The drawing under review shows one solid part. Ordinate dimensions are in mm from its lowest x, y, z. Coordinates: 2 decimals unless noted, no trailing zeros. Write each loop counter-clockwise with the first axis right and the second up, starting at its lowest first coordinate (ties: lowest second). Pieces come first, ordered by that corner, then holes.
Q1. Add section B-B, the plane y = 81.5. Give the boundary of the cut face in (x, z), plus the area to 3 significant figures.
Q2. Add section A-A, the plane x = 61.5. Give the boundary of the cut face in (y, z).
Q3. The part is to be moulded in two halves that separate along Y. For the marked faces 1, 2 and 3, say which applies: +Y half, -Y half, draft (parallel to the pull), parting line (faces both ways), or undercut.
Q4. Add section C-C, the plane x = 92. Give the boundary of the cut face in (y, z) (1 decimal).
Q5. To check wall thickness, follow probe 1 along Y at (x, z) = (61.5, 7.55); probe 2 along X at (y, z) = (52.5, 1) (1 decimal); probe 3 along X at (y, z) = (23, 5.5) (1 decimal). State the ranges of each line that lie inside material, in increasing order.
Q6. Clearance check with flat-ended pins moving along their axes: pin 1 Ø2.5 at (x, y) = (61.5, 6) entering from +Z; pin 2 Ø4.5 at (y, z) = (62, 2.5) entering from -X; pin 3 Ø1 at (y, z) = (86, 1) entering from +X; pin 4 Ø5 at (y, z) = (94.5, 3) entering from +X (1 decimal). State where each tip first meets the part, or that it passes through.
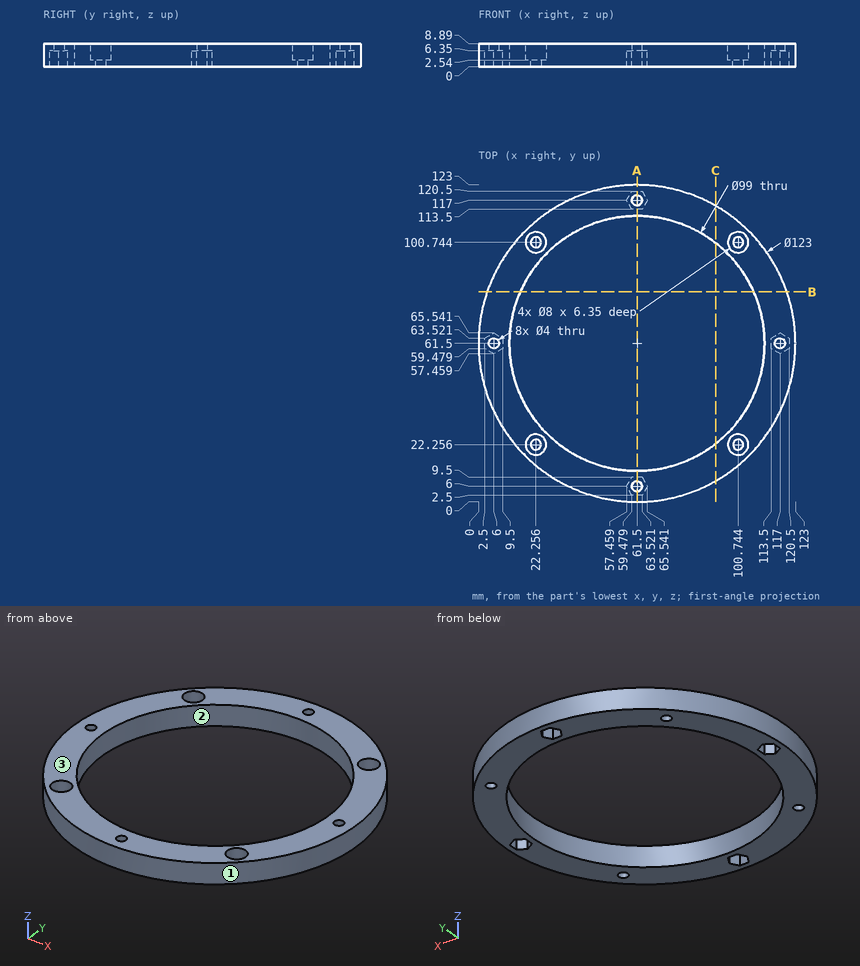
Here are the results:
1. outline: (3.34, 0) - (16.22, 0) - (16.22, 8.89) - (3.34, 8.89) - close; (106.78, 0) - (119.66, 0) - (119.66, 8.89) - (106.78, 8.89) - close
1. area: 229 mm2
2. outline: (0, 0) - (2.5, 0) - (2.5, 6.35) - (4, 6.35) - (4, 8.89) - (0, 8.89) - close; (8, 6.35) - (9.5, 6.35) - (9.5, 0) - (12, 0) - (12, 8.89) - (8, 8.89) - close; (111, 0) - (113.5, 0) - (113.5, 6.35) - (115, 6.35) - (115, 8.89) - (111, 8.89) - close; (119, 6.35) - (120.5, 6.35) - (120.5, 0) - (123, 0) - (123, 8.89) - (119, 8.89) - close
3. face 1: parting line
3. face 2: undercut
3. face 3: draft
4. outline: (8.1, 0) - (22.5, 0) - (22.5, 8.9) - (8.1, 8.9) - close; (100.5, 0) - (114.9, 0) - (114.9, 8.9) - (100.5, 8.9) - close
5. probe 1: y = 0 to 4, 8 to 12, 111 to 115, 119 to 123
5. probe 2: x = 0.7 to 12.8, 110.2 to 122.3
5. probe 3: x = 13.5 to 18.3, 26.2 to 30.4, 92.6 to 96.8, 104.7 to 109.5
6. pin 1: passes through
6. pin 2: stops at x = 0
6. pin 3: stops at x = 118.12
6. pin 4: stops at x = 114.9
